Geometry check sheet. Reference: the model listing, model coordinates, mm. A direction names the side the tool comes from. Coordinates: 2 decimals unless noted, no trailing zeros. Write each loop counter-clockwise with the first axis right and the second up, starting at its lowest first coordinate (ties: lowest second). Pieces come first, ordered by that corner, then holes. Notation, with made-up numbers: (-27, 70) -> (32, 70) arc R16 ccw to (32, 95) -> close; hole circle Ø8 at (17.5, 50). An arc over 180 degrees is marked (long way). Use a Markdown table: item, result.
```python
from build123d import *

# Parameters (mm, degrees)
BOSS_EXTRUDE2_DEPTH = 215.9
SKETCH5_OUTSIDE_W   = 51.574
SKETCH5_OUTSIDE_H   = 52.556
SKETCH5_OUTSIDE_R   = 3.175
CUT_EXTRUDE1_DEPTH  = 12.7
SKETCH6_OUTSIDE_W   = 51.574
SKETCH6_OUTSIDE_H   = 52.556
SKETCH6_OUTSIDE_R   = 3.175
CUT_EXTRUDE2_DEPTH  = 12.7
SKETCH7_OUTSIDE_W   = 51.574
SKETCH7_OUTSIDE_H   = 52.556
SKETCH7_OUTSIDE_R   = 2.667
CUT_EXTRUDE3_DEPTH  = 0.762
SKETCH9_OUTSIDE_W   = 51.574
SKETCH9_OUTSIDE_H   = 52.556
SKETCH9_OUTSIDE_R   = 2.667
CUT_EXTRUDE4_DEPTH  = 0.762


with BuildPart() as part:
    # Sketch3 → Boss-Extrude2 (new body)
    with BuildSketch(Plane.XY):
        Polygon((0, 3.666174209), (-3.175, 1.833087105), (-3.175, -1.833087105), (0, -3.666174209), (3.175, -1.833087105), (3.175, 1.833087105), align=None)
    extrude(amount=BOSS_EXTRUDE2_DEPTH)

    # Sketch5 outside → Cut-Extrude1 (cut)
    with BuildSketch(Plane(origin=(0, 0, 0), x_dir=(-1, 0, 0), z_dir=(0, 0, -1))):
        Rectangle(SKETCH5_OUTSIDE_W, SKETCH5_OUTSIDE_H)
        with Locations(Location((0, 0, 0), (0, 0, 180))):
            Circle(SKETCH5_OUTSIDE_R, mode=Mode.SUBTRACT)
    extrude(amount=-CUT_EXTRUDE1_DEPTH, mode=Mode.SUBTRACT)

    # Sketch6 outside → Cut-Extrude2 (cut)
    with BuildSketch(Plane.XY.offset(215.9)):
        Rectangle(SKETCH6_OUTSIDE_W, SKETCH6_OUTSIDE_H)
        Circle(SKETCH6_OUTSIDE_R, mode=Mode.SUBTRACT)
    extrude(amount=-CUT_EXTRUDE2_DEPTH, mode=Mode.SUBTRACT)

    # Sketch7 outside → Cut-Extrude3 (cut)
    with BuildSketch(Plane.XY.offset(214.63)):
        Rectangle(SKETCH7_OUTSIDE_W, SKETCH7_OUTSIDE_H)
        Circle(SKETCH7_OUTSIDE_R, mode=Mode.SUBTRACT)
    extrude(amount=-CUT_EXTRUDE3_DEPTH, mode=Mode.SUBTRACT)

    # Sketch9 outside → Cut-Extrude4 (cut)
    with BuildSketch(Plane(origin=(0, 0, 1.27), x_dir=(-1, 0, 0), z_dir=(0, 0, -1))):
        Rectangle(SKETCH9_OUTSIDE_W, SKETCH9_OUTSIDE_H)
        with Locations(Location((0, 0, 0), (0, 0, 180))):
            Circle(SKETCH9_OUTSIDE_R, mode=Mode.SUBTRACT)
    extrude(amount=-CUT_EXTRUDE4_DEPTH, mode=Mode.SUBTRACT)


solid = part.part
```
Item 1: Thickness scan on L1, parallel to Z at x = 2.75, y = 1; L2, parallel to X at y = 2.75, z = 43; L3, parallel to Z at x = 2.75, y = 1.75. Record the ranges inside material, lowest first. Write a range as [from, to].
Answer block:
| item | result |
|---|---|
| L1 | z = [0, 1.27], [2.03, 213.87], [214.63, 215.9] |
| L2 | x = [-1.59, 1.59] |
| L3 | z = [12.7, 203.2] |
Item 2: Depth check by flat-ended pin: P1, Ø1, axis at x = 2, z = 178.5, coming from the -Y side; P2, Ø0.5, axis at x = 0, y = -3, coming from the -Z side. Enter the tip coordinate at first touch or a pass-through.
Answer block:
| item | result |
|---|---|
| P1 | stops at y = -2.8 |
| P2 | stops at z = 0 |
Item 3: Tool access check on faces 1 (the cylindrical face through (1.5, 2.8, 0.6)), 2 (the cylindrical face through (1.231, 2.366, 1.646)), 3 (the flat face through (-3.175, 0, 107)), 4 (the cylindrical face through (-0.69, -3.1, 215.27)). Record the directions out of +Z, -Z, +X, -X, +Y, -Y that give a thin tool (end or side, any length) a straight path to the whole face; none if there is none.
Answer block:
| item | result |
|---|---|
| face 1 | -Z |
| face 2 | none |
| face 3 | +Z, -Z, -X, +Y, -Y |
| face 4 | +Z |
Item 4: Section check A-A on z = 136. Record the boundary of the cut face in (x, y) (3 decimals), then the cut area to 3 significant figures.
Answer block:
| item | result |
|---|---|
| outline | (-3.175, -1.833) -> (0, -3.666) -> (3.175, -1.833) -> (3.175, 1.833) -> (0, 3.666) -> (-3.175, 1.833) -> close |
| area | 34.9 mm^2 |
Item 5: Mould release check, pull along Z, two halves, no side actions. Record for faces 5 (the flat face through (0, 0, 215.9)), 6 (the cylindrical face through (-0.69, -3.1, 208.61)), 7 (the flat face through (-2, 2, 214.63)): +Z half, -Z half, draft (parallel to the pull), parting line (faces both ways), or undercut.
Answer block:
| item | result |
|---|---|
| face 5 | +Z half |
| face 6 | draft |
| face 7 | undercut |
